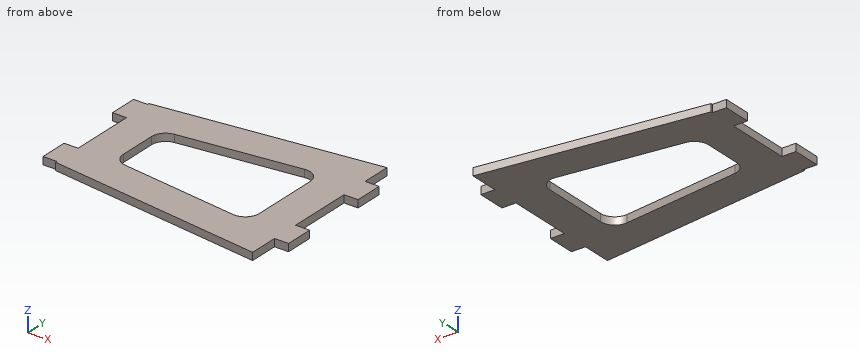
from build123d import *

# Parameters (mm, degrees)
BOSS_EXTRUDE1_DEPTH = 3.4036


with BuildPart() as part:
    # Sketch1 → Boss-Extrude1 (new body)
    with BuildSketch(Plane.XY):
        Polygon((8672.177263948, 2928.441804612), (8678.527263948, 2928.441804612), (8678.527263948, 2941.141804612), (8672.177263948, 2941.141804612), (8672.177263948, 2970.351804612), (8678.527263948, 2970.351804612), (8678.527263948, 2983.051804612), (8672.177263948, 2983.051804612), (8672.177263948, 2996.259804612), (8573.879263948, 2983.853260922), (8573.879263948, 2983.051804612), (8567.529263948, 2983.051804612), (8567.529263948, 2970.351804612), (8573.879263948, 2970.351804612), (8573.879263948, 2941.141804612), (8567.529263948, 2941.141804612), (8567.529263948, 2928.441804612), (8573.879263948, 2928.441804612), (8573.879263948, 2927.640348301), (8672.177263948, 2915.233804612), align=None)
        with BuildLine():
            Line((8589.754263948, 2964.257036739), (8589.754263948, 2947.236572484))
            ThreePointArc((8589.754263948, 2947.236572484), (8591.34129796, 2943.036970717), (8595.309115917, 2940.936553468))
            Line((8595.309115917, 2940.936553468), (8649.157115917, 2934.140203953))
            ThreePointArc((8649.157115917, 2934.140203953), (8654.151865715, 2935.677256982), (8656.302263948, 2940.44022297))
            Line((8656.302263948, 2940.44022297), (8656.302263948, 2971.053386254))
            ThreePointArc((8656.302263948, 2971.053386254), (8654.151865715, 2975.816352241), (8649.157115917, 2977.35340527))
            Line((8649.157115917, 2977.35340527), (8595.309115917, 2970.557055756))
            ThreePointArc((8595.309115917, 2970.557055756), (8591.34129796, 2968.456638506), (8589.754263948, 2964.257036739))
        make_face(mode=Mode.SUBTRACT)
    extrude(amount=BOSS_EXTRUDE1_DEPTH)


solid = part.part
Verification items for the finished model (mm, model axes). Give positions to 0.01 mm unless a question says otherwise; leave off trailing zeros. Order: outer loops, then holes, each group sorted by start corner. A loop starts at its lowest first (then second) coordinate and runs counter-clockwise, first axis right, second up. Notation, with made-up numbers: (45.25, 57) -> (85.25, 57) arc R13 cw to (85.25, 79) -> close; hole circle Ø6 at (20, 87). An arc over 180 degrees is marked (long way). Answer as CSV lines item,"result".
Q1. Sectioned sample at B-B on x = 8643. Record the cut outline in (y, z).
Solutions:
outline,"(2918.92, 0) -> (2934.92, 0) -> (2934.92, 3.4) -> (2918.92, 3.4) -> close; (2976.58, 0) -> (2992.58, 0) -> (2992.58, 3.4) -> (2976.58, 3.4) -> close"
Q2. Sectioned sample at D-D on x = 8580. Record the cut outline in (y, z), plus the area to 3 significant figures.
Solutions:
outline,"(2926.87, 0) -> (2984.63, 0) -> (2984.63, 3.4) -> (2926.87, 3.4) -> close"
area,"197 mm²"
Q3. Depth check by flat-ended pin: pin 1 (1.7 mm diameter, centred on x = 8572, z = 1, fed in from -Y); pin 2 (1.5 mm diameter, centred on x = 8666, z = 2, fed in from -Y); pin 3 (1 mm diameter, centred on y = 2962.5, z = 2, fed in from -X). Enter the tip coordinate at first touch or a pass-through.
Solutions:
pin 1,"stops at y = 2928.44"
pin 2,"stops at y = 2915.92"
pin 3,"stops at x = 8573.88"
Q4. Sectioned sample at A-A on y = 2966. Record the cut outline in (x, z), plus the area to 3 significant figures.
Solutions:
outline,"(8573.88, 0) -> (8590, 0) -> (8590, 3.4) -> (8573.88, 3.4) -> close; (8656.3, 0) -> (8672.18, 0) -> (8672.18, 3.4) -> (8656.3, 3.4) -> close"
area,"109 mm²"
Q5. Sectioned sample at C-C on z = 2.6. Record the cut outline in (x, y).
Solutions:
outline,"(8567.53, 2928.44) -> (8573.88, 2928.44) -> (8573.88, 2927.64) -> (8672.18, 2915.23) -> (8672.18, 2928.44) -> (8678.53, 2928.44) -> (8678.53, 2941.14) -> (8672.18, 2941.14) -> (8672.18, 2970.35) -> (8678.53, 2970.35) -> (8678.53, 2983.05) -> (8672.18, 2983.05) -> (8672.18, 2996.26) -> (8573.88, 2983.85) -> (8573.88, 2983.05) -> (8567.53, 2983.05) -> (8567.53, 2970.35) -> (8573.88, 2970.35) -> (8573.88, 2941.14) -> (8567.53, 2941.14) -> close; hole (8589.75, 2947.24) arc R6.35 ccw to (8595.31, 2940.94) -> (8649.16, 2934.14) arc R6.35 ccw to (8656.3, 2940.44) -> (8656.3, 2971.05) arc R6.35 ccw to (8649.16, 2977.35) -> (8595.31, 2970.56) arc R6.35 ccw to (8589.75, 2964.26) -> close"
Q6. Scan lines: probe 1 along X at (y, z) = (2947, 2.95); probe 2 along Y at (x, z) = (8644, 2.6); probe 3 along Y at (x, z) = (8643.5, 1.15). Record each from-to range of solid material in increasing order.
Solutions:
probe 1,"x = 8573.88 to 8589.76, 8656.3 to 8672.18"
probe 2,"y = 2918.79 to 2934.79, 2976.7 to 2992.7"
probe 3,"y = 2918.85 to 2934.85, 2976.64 to 2992.64"
